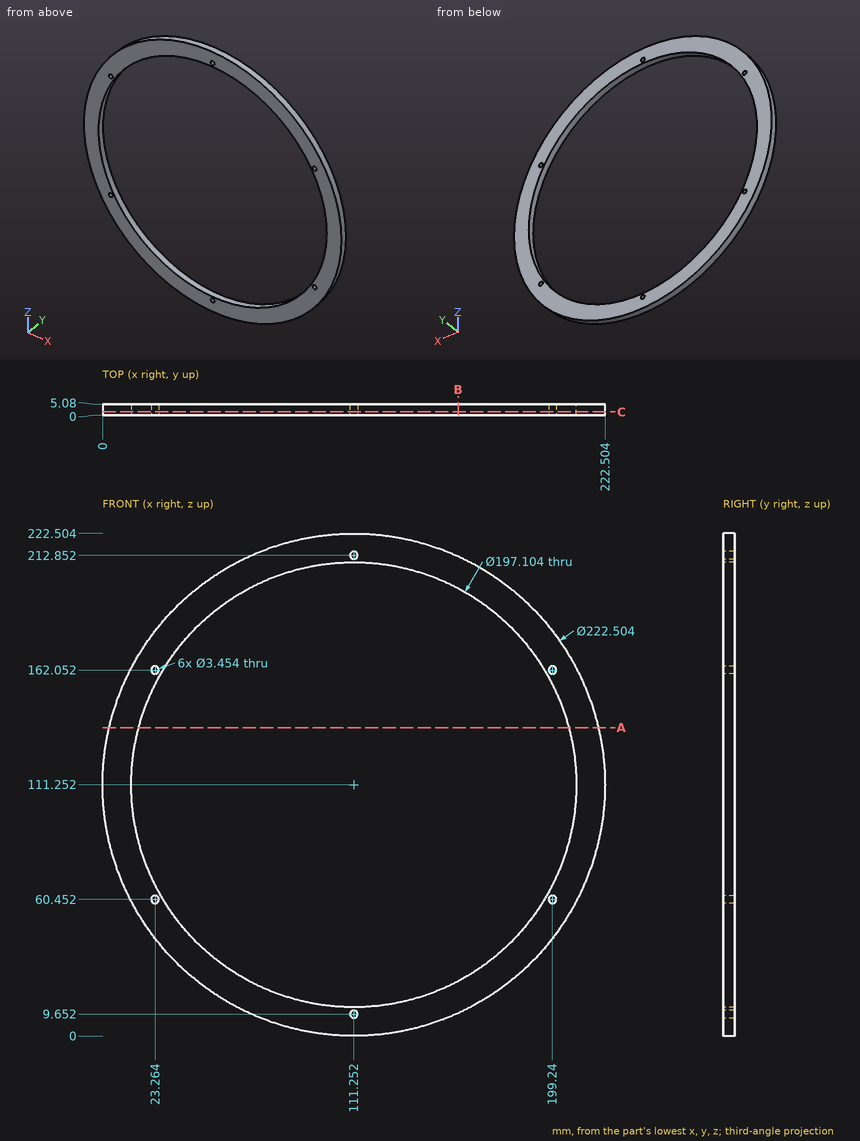
Could you check a few things on this drawing? It's one solid part, dimensions in mm from its lowest x, y, z. Coordinates: 2 decimals unless noted, no trailing zeros. Loops run counter-clockwise (first coordinate to the right, second up) from the corner with the lowest first, then second, coordinate; pieces in that order, holes last.
1. I need wall thicknesses on L1, parallel to X at y = 3.55, z = 161 (1 decimal); L2, parallel to Z at x = 22.5, y = 2.4 (1 decimal); L3, parallel to Z at x = 105.5, y = 0.95 (1 decimal). Which ranges of each line are inside material? Lowest first, please.
2. Imagine slicing it at A-A (z = 136.5). Please give me the cut outline in (x, y) (1 decimal), and give its area (3 significant figures).
3. Imagine slicing it at B-B (x = 157.5). Please give me the cut outline in (y, z) (1 decimal), and give its area (3 significant figures).
4. For P1, Ø3, axis at x = 134, y = 4, coming from the +Z side; P2, Ø3, axis at y = 3.5, z = 118, coming from the +X side, each with a flat end and sliding along its axis, tell me the tip position at first contact or that it passes through.
5. Imagine slicing it at C-C (y = 1.6). Please give me the cut outline in (x, z) (1 decimal).
Computed values:
1. L1: x = 11.7 to 21.9, 24.6 to 26.2, 196.3 to 197.9, 200.6 to 210.8
1. L2: z = 44.2 to 58.9, 62 to 68.4, 154.1 to 160.5, 163.6 to 178.3
1. L3: z = 0.1 to 12.9, 209.6 to 222.4
2. outline: (2.9, 0) - (16, 0) - (16, 5.1) - (2.9, 5.1) - close; (206.5, 0) - (219.6, 0) - (219.6, 5.1) - (206.5, 5.1) - close
2. area: 133 mm2
3. outline: (0, 10.1) - (5.1, 10.1) - (5.1, 24.2) - (0, 24.2) - close; (0, 198.3) - (5.1, 198.3) - (5.1, 212.4) - (0, 212.4) - close
3. area: 144 mm2
4. P1: stops at z = 220.46
4. P2: stops at x = 222.38
5. outline: circle Ø222.5 at (111.3, 111.3); hole circle Ø197.1 at (111.3, 111.3); hole circle Ø3.5 at (23.3, 60.5); hole circle Ø3.5 at (23.3, 162.1); hole circle Ø3.5 at (111.3, 9.7); hole circle Ø3.5 at (111.3, 212.9); hole circle Ø3.5 at (199.2, 60.5); hole circle Ø3.5 at (199.2, 162.1)
